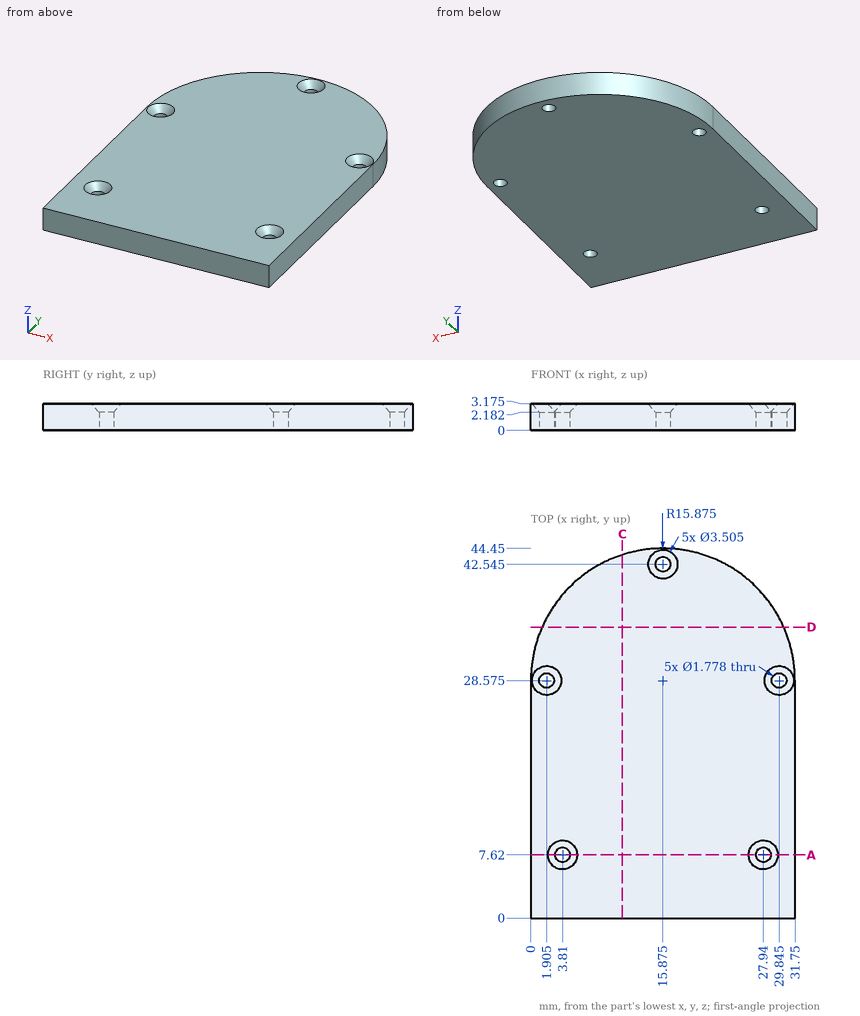
Geometry: see drawing. Coordinates: mm, zero at the bounding-box minimum. Round coordinates to 2 decimals unless told otherwise and drop trailing zeros. Loops run counter-clockwise (first coordinate to the right, second up) from the corner with the lowest first, then second, coordinate; pieces in that order, holes last. Notation, with made-up numbers: (18, 32) -> (43, 32) arc R17 cw to (43, 40) -> close; hole circle Ø5 at (51, 57). An arc over 180 degrees is marked (long way). Write each question's results on one line, items separated by ' | '.
Item 1: Cut plane D-D on y = 35. Return the cut outline in (x, z) (1 decimal).
Answers below:
outline: (1.4, 0) -> (30.4, 0) -> (30.4, 3.2) -> (1.4, 3.2) -> close
Item 2: Cut plane C-C on x = 11. Return the cut outline in (y, z) (1 decimal).
Answers below:
outline: (0, 0) -> (43.7, 0) -> (43.7, 3.2) -> (0, 3.2) -> close
Item 3: Pin query (flat end, axial travel): pin 1 Ø1.5 at (x, z) = (14.5, 0.5) entering from +Y; pin 2 Ø1 at (x, z) = (13.5, 1) entering from +Y; pin 3 Ø1.5 at (y, z) = (30.5, 2) entering from +X. Return the tip coordinate at first contact, or that it passes through.
Answers below:
pin 1: stops at y = 44.44 | pin 2: stops at y = 44.34 | pin 3: stops at x = 31.71
Item 4: Line query: probe 1 along Y at (x, z) = (29, 2.75) (1 decimal); probe 2 along Y at (x, z) = (27.94, 1.25) (1 decimal); probe 3 along Y at (x, z) = (3, 2.25) (1 decimal). Output: solid intervals per line, ascending. Write a range as [from, to].
Answers below:
probe 1: y = [0, 6.7], [8.5, 27.5], [29.7, 37.5] | probe 2: y = [0, 6.7], [8.5, 38.9] | probe 3: y = [0, 7.1], [8.1, 37.9]
Item 5: Cut plane A-A on y = 7.62. State how many separate pieces and enclosed holes the cut face has.
Answers below:
separate pieces: 3 | enclosed holes: 0
